```python
from build123d import *

# Parameters (mm, degrees)
F0_R     = 3
F0_R_2   = 5.5
F1_DEPTH = 8
F2_R     = 18


with BuildPart() as f1:
    # F0 (on Top) → F1 (new body)
    with BuildSketch(Plane.XY):
        with BuildLine():
            ThreePointArc((8.685422, 70.970583), (2.590905, 68.894208), (0, 63))
            Line((0, 63), (0, 8))
            ThreePointArc((0, 8), (2.343146, 2.343146), (8, 0))
            Line((8, 0), (93, 0))
            ThreePointArc((93, 0), (104.702957, 9.346551), (98.175532, 22.826535))
            Line((98.175532, 22.826535), (61.6736, 40.275971))
            Line((61.6736, 40.275971), (43.620393, 62.728427))
            Line((43.620393, 62.728427), (8.685422, 70.970583))
        make_face()
        with Locations((8, 8)):
            Circle(F0_R, mode=Mode.SUBTRACT)
        with BuildLine():
            Line((17, 21), (17, 39.730763))
            ThreePointArc((17, 39.730763), (18.86701, 43.1146), (22.725177, 43.339608))
            Line((22.725177, 43.339608), (28.013733, 40.811459))
            Line((28.013733, 40.811459), (30.749989, 46.535348))
            ThreePointArc((30.749989, 46.535348), (36.084011, 48.419016), (37.967679, 43.084993))
            Line((37.967679, 43.084993), (35.231423, 37.361104))
            Line((35.231423, 37.361104), (61.907477, 24.608845))
            ThreePointArc((61.907477, 24.608845), (64.083285, 20.115517), (60.182299, 17))
            Line((60.182299, 17), (21, 17))
            ThreePointArc((21, 17), (18.171573, 18.171573), (17, 21))
        make_face(mode=Mode.SUBTRACT)
        with Locations((93, 12)):
            Circle(F0_R_2, mode=Mode.SUBTRACT)
        with Locations((8, 63)):
            Circle(F0_R, mode=Mode.SUBTRACT)
    extrude(amount=F1_DEPTH)

    # F2
    f2_edges = [f1.edges().sort_by_distance(p)[0] for p in [
        (43.620393, 62.728427, 4),
        (61.6736, 40.275971, 4),
    ]]
    fillet(f2_edges, radius=F2_R)


solid = f1.part
```
Check sheet for the modelled part. Datum: model origin and axes. Units: mm. A direction names the side the tool comes from. Coordinates: 2 decimals unless noted, no trailing zeros. Write each loop counter-clockwise with the first axis right and the second up, starting at its lowest first coordinate (ties: lowest second). Pieces come first, ordered by that corner, then holes. Notation, with made-up numbers: (76, 56.25) -> (94, 56.25) arc R16 ccw to (94, 73.25) -> close; hole circle Ø11 at (-31.75, 52). An arc over 180 degrees is marked (long way). Use a Markdown table: item, result.
1. Scan lines: line 1 along Y through (x, z) = (8, 6); line 2 along Y through (x, z) = (10, 0.75); line 3 along X through (y, z) = (10.5, 7). Record each from-to range of solid material in increasing order.
Reported:
| item | result |
|---|---|
| line 1 | y = 0 to 5, 11 to 60, 66 to 71 |
| line 2 | y = 0 to 5.76, 10.24 to 60.76, 65.24 to 70.66 |
| line 3 | x = 0 to 6.34, 9.66 to 87.71, 98.29 to 104.91 |
2. Sectioned sample at B-B (x = 90). Enter the section's corners in (y, z).
Reported:
| item | result |
|---|---|
| outline | (0, 0) -> (7.39, 0) -> (7.39, 8) -> (0, 8) -> close; (16.61, 0) -> (26.73, 0) -> (26.73, 8) -> (16.61, 8) -> close |
3. Tool access check on faces 4 (the flat face through (17, 30, 4)), 5 (the flat face through (40, 36, 8)). Record the directions out of +Z, -Z, +X, -X, +Y, -Y that give a thin tool (end or side, any length) a straight path to the whole face; none if there is none.
Reported:
| item | result |
|---|---|
| face 4 | +Z, -Z |
| face 5 | +Z, +X, -X, +Y, -Y |
4. Release check for a two-part mould opening along Y. For faces 1 (the cylindrical face through (18.203, 18.141, 3.944)), 2 (the flat face through (40, 36, 0)), 3 (the flat face through (23.35, 67.51, 3.94)) record: pulls with the +Y half, pulls with the -Y half, needs draft (parallel to the pull), parting line crosses it, or undercut.
Reported:
| item | result |
|---|---|
| face 1 | undercut |
| face 2 | needs draft |
| face 3 | pulls with the +Y half |
5. Sectioned sample at D-D (x = 6.5). Enter the section's corners in (y, z).
Reported:
| item | result |
|---|---|
| outline | (0.14, 0) -> (5.4, 0) -> (5.4, 8) -> (0.14, 8) -> close; (10.6, 0) -> (60.4, 0) -> (60.4, 8) -> (10.6, 8) -> close; (65.6, 0) -> (70.86, 0) -> (70.86, 8) -> (65.6, 8) -> close |
6. Sectioned sample at A-A (z = 4.25). Enter the section's corners in (x, y) (1 decimal), plus the area to 3 significant figures.
Reported:
| item | result |
|---|---|
| outline | (0, 8) arc R8 ccw to (8, 0) -> (93, 0) arc R12 ccw to (98.2, 22.8) -> (65.4, 38.5) arc R18 cw to (59.1, 43.5) -> (47.5, 57.9) arc R18 ccw to (37.6, 64.1) -> (8.7, 71) arc R8 ccw to (0, 63) -> close; hole circle Ø6 at (8, 8); hole circle Ø6 at (8, 63); hole (17, 21) arc R4 ccw to (21, 17) -> (60.2, 17) arc R4 ccw to (61.9, 24.6) -> (35.2, 37.4) -> (38, 43.1) arc R4 ccw to (30.7, 46.5) -> (28, 40.8) -> (22.7, 43.3) arc R4 ccw to (17, 39.7) -> close; hole circle Ø11 at (93, 12) |
| area | 4,060 mm2 |
7. Sectioned sample at C-C (y = 14). Enter the section's corners in (x, z).
Reported:
| item | result |
|---|---|
| outline | (0, 0) -> (87.88, 0) -> (87.88, 8) -> (0, 8) -> close; (98.12, 0) -> (104.83, 0) -> (104.83, 8) -> (98.12, 8) -> close |
8. Go/stop test with a flat-tipped pin: pin 1 Ø5.5 at (x, y) = (8, 8) entering from +Z. Record where the tip stops, or that it passes through.
Reported:
| item | result |
|---|---|
| pin 1 | passes through |
